Design review of the part built by this model. Coordinates are the model's own, in mm. A direction names the side the tool comes from. Coordinates: 2 decimals unless noted, no trailing zeros. Write each loop counter-clockwise with the first axis right and the second up, starting at its lowest first coordinate (ties: lowest second). Pieces come first, ordered by that corner, then holes. Notation, with made-up numbers: M 79.25,41.25 L 137.25,41.25 A26 ccw 137.25,74.25 Z; hole C -11,33.25 d3. An arc over 180 degrees is marked long. Write item = value, one per line.
```python
from build123d import *

# Parameters (mm, degrees)
DODANIE_WYCI_GNI_CIE1_DEPTH = 40
WYTNIJ_WYCI_GNI_CIE1_REACH  = 72.711
SZKIC2_R                    = 6.5
SFAZOWANIE1_SIZE            = 2
ZAOKR_GLENIE1_R             = 2


with BuildPart() as part:
    # Szkic1 → Dodanie-wyciągnięcie1 (new body)
    with BuildSketch(Plane.XY):
        with BuildLine():
            Line((50, 0), (20, 0))
            ThreePointArc((20, 0), (0, -20), (-20, 0))
            Line((-20, 0), (-50, 0))
            Line((-50, 0), (-50, -30))
            Line((-50, -30), (50, -30))
            Line((50, -30), (50, 0))
        make_face()
    extrude(amount=DODANIE_WYCI_GNI_CIE1_DEPTH)

    # Szkic2 → Wytnij-wyciągnięcie1 (cut, up to next)
    with BuildSketch(Plane(origin=(0, 0, 0), x_dir=(1, 0, 0), z_dir=(0, 1, 0)), mode=Mode.PRIVATE) as wytnij_wyci_gni_cie1_sk1:
        with Locations(Location((-35, -20, 0), (0, 0, 270))):
            Circle(SZKIC2_R)
    wytnij_wyci_gni_cie1_tool1 = extrude(wytnij_wyci_gni_cie1_sk1.sketch, amount=-WYTNIJ_WYCI_GNI_CIE1_REACH, mode=Mode.PRIVATE) & part.part
    # Szkic2 → Wytnij-wyciągnięcie1 (cut, up to next)
    with BuildSketch(Plane(origin=(0, 0, 0), x_dir=(1, 0, 0), z_dir=(0, 1, 0)), mode=Mode.PRIVATE) as wytnij_wyci_gni_cie1_sk2:
        with Locations(Location((35, -20, 0), (0, 0, 270))):
            Circle(SZKIC2_R)
    wytnij_wyci_gni_cie1_tool2 = extrude(wytnij_wyci_gni_cie1_sk2.sketch, amount=-WYTNIJ_WYCI_GNI_CIE1_REACH, mode=Mode.PRIVATE) & part.part
    add(wytnij_wyci_gni_cie1_tool1.solids().sort_by_distance((-35, 0, 20))[0], mode=Mode.SUBTRACT)
    add(wytnij_wyci_gni_cie1_tool2.solids().sort_by_distance((35, 0, 20))[0], mode=Mode.SUBTRACT)

    # Sfazowanie1
    sfazowanie1_edges = [part.edges().sort_by_distance(p)[0] for p in [
        (-35, 0, 13.5),
        (-35, -30, 13.5),
        (35, 0, 13.5),
        (35, -30, 13.5),
    ]]
    chamfer(sfazowanie1_edges, length=SFAZOWANIE1_SIZE)

    # Zaokrąglenie1
    zaokr_glenie1_edges = [part.edges().sort_by_distance(p)[0] for p in [
        (0, -20, 0),
        (-35, 0, 40),
        (20, 0, 20),
        (50, 0, 20),
        (50, -30, 20),
        (-50, -30, 20),
        (-50, 0, 20),
        (-20, 0, 20),
        (-50, -15, 40),
        (0, -30, 40),
        (50, -15, 40),
        (35, 0, 40),
        (0, -20, 40),
        (35, 0, 0),
        (50, -15, 0),
        (0, -30, 0),
        (-50, -15, 0),
        (-35, 0, 0),
    ]]
    fillet(zaokr_glenie1_edges, radius=ZAOKR_GLENIE1_R)


solid = part.part
```
Q1. Wall thickness on line 1 (X direction, y = -20.5, z = 20); line 2 (X direction, y = -9.5, z = 20); line 3 (X direction, y = -3.5, z = 19.5): over which ranges is each line inside the solid? List them lowest first.
Check result:
line_1 = -50 to -41.5, -28.5 to 28.5, 41.5 to 50
line_2 = -50 to -41.5, -28.5 to -17.6, 17.6 to 28.5, 41.5 to 50
line_3 = -50 to -41.48, -28.52 to -19.69, 19.69 to 28.52, 41.48 to 50
Q2. Consider section C-C, the plane x = 35. State the section outline as (y, z) points.
Check result:
outline = M -30,2 A2 ccw -28,0 L -2,0 A2 ccw 0,2 L 0,11.5 L -2,13.5 L -28,13.5 L -30,11.5 Z; M -30,28.5 L -28,26.5 L -2,26.5 L 0,28.5 L 0,38 A2 ccw -2,40 L -28,40 A2 ccw -30,38 Z
Q3. Consider section D-D, the plane z = 7.5. State the section outline as (x, y) points.
Check result:
outline = M -50,-28 A2 ccw -48,-30 L 48,-30 A2 ccw 50,-28 L 50,-2 A2 ccw 48,0 L 21.91,0 A2 ccw 19.92,-1.82 A20 cw -19.92,-1.82 A2 ccw -21.91,0 L -48,0 A2 ccw -50,-2 Z
Q4. Consider section A-A, the plane z = 20. State the section outline as (x, y) points.
Check result:
outline = M -50,-28 A2 ccw -48,-30 L -43.5,-30 L -41.5,-28 L -41.5,-2 L -43.5,0 L -48,0 A2 ccw -50,-2 Z; M -28.5,-28 L -26.5,-30 L 26.5,-30 L 28.5,-28 L 28.5,-2 L 26.5,0 L 21.91,0 A2 ccw 19.92,-1.82 A20 cw -19.92,-1.82 A2 ccw -21.91,0 L -26.5,0 L -28.5,-2 Z; M 41.5,-28 L 43.5,-30 L 48,-30 A2 ccw 50,-28 L 50,-2 A2 ccw 48,0 L 43.5,0 L 41.5,-2 Z
Q5. Consider section B-B, the plane y = -23.75. State the section outline as (x, z) points, and give its area (3 significant figures).
Check result:
outline = M -50,2 A2 ccw -48,0 L 48,0 A2 ccw 50,2 L 50,38 A2 ccw 48,40 L -48,40 A2 ccw -50,38 Z; hole C -35,20 d13; hole C 35,20 d13
area = 3,730 mm²
Q6. Machinability: for faces 1 (the cylindrical face through (20.576, -0.509, 20.252)), 2 (the cylindrical face through (0.67, -29.4, 0.57)), which of the approach directions +Z, -Z, +X, -X, +Y, -Y give a long, thin tool a straight path to every point of the face, cutting with its end or side? Answer none if there is none.
Check result:
face_1 = +Z, -Z, +Y
face_2 = -Z, +X, -X, -Y
Q7. The part is to be moulded in two halves that separate along Z. For faces 3 (the cylindrical face through (-30.607, -14.818, 15.209)), 4 (the conical face through (41.569, -28.125, 19.138)), 5 (the cylindrical face through (-35.14, -0.6, 0.57)), 6 (the cylindrical face through (-20.545, -0.537, 20.252)), say which applies: +Z half, -Z half, draft (parallel to the pull), parting line (faces both ways), or undercut.
Check result:
face_3 = undercut
face_4 = undercut
face_5 = -Z half
face_6 = draft
Q8. For P1, Ø3, axis at x = 12.5, y = -15, coming from the -Z side; P2, Ø6, axis at x = -19, z = 35.5, coming from the +Y side; P3, Ø3, axis at x = 0, z = 23.5, coming from the +Y side, all flat-tipped, find the tip position at first contact; note any pin that passes through.
Check result:
P1 = 0.25
P2 = 0
P3 = -19.94
